Read the model definition and answer for the solid it produces. Units are mm, in the model's axes. Face numbers are marked on the shaded views. A direction names the side the tool comes from. Give positions to 0.01 mm unless a question says otherwise; leave off trailing zeros. Loops run counter-clockwise (first coordinate to the right, second up) from the corner with the lowest first, then second, coordinate; pieces in that order, holes last. Notation, with made-up numbers: (-21, -9) - (28, -9) arc R24 cw to (28, 28) - close; hole circle Ø1 at (74, 85). An arc over 180 degrees is marked (long way). Write item = value, one per line.
```python
from build123d import *

# Parameters (mm, degrees)
SKETCH_2_OUTSIDE_W       = 102.04
SKETCH_2_OUTSIDE_H       = 102.04
SKETCH_2_OUTSIDE_W_2     = 32
SKETCH_2_OUTSIDE_H_2     = 32
CUT_EXTRUDE_1_DEPTH      = 24
CUT_EXTRUDE_2_DEPTH      = 5
CUT_EXTRUDE_3_DEPTH      = 243.590189414
CUT_EXTRUDE_3_DEPTH_BACK = 243.590189414
SKETCH_4_R               = 6


with BuildPart() as part:
    # Эскиз1 → Повернуть1 (revolve)
    with BuildSketch(Plane.XY, mode=Mode.PRIVATE) as revolve_1_sk:
        Polygon((0, 0), (0, 19), (-1, 20), (-160, 20), (-160, 25), (-184, 25), (-184, 16), (-239, 16), (-240, 15), (-240, 0), align=None)
    revolve(revolve_1_sk.sketch.rotate(Axis((-178.322580645, 0, 0), (1, 0, 0)), 90), axis=Axis((-178.322580645, 0, 0), (1, 0, 0)))

    # Эскиз2 outside → Вырез-Вытянуть1 (cut)
    with BuildSketch(Plane(origin=(-144, 0, 0), x_dir=(0, 0, -1), z_dir=(1, 0, 0))):
        Rectangle(SKETCH_2_OUTSIDE_W, SKETCH_2_OUTSIDE_H)
        Rectangle(SKETCH_2_OUTSIDE_W_2, SKETCH_2_OUTSIDE_H_2, mode=Mode.SUBTRACT)
    extrude(amount=CUT_EXTRUDE_1_DEPTH, mode=Mode.SUBTRACT)

    # Эскиз3 → Вырез-Вытянуть2 (cut)
    with BuildSketch(Plane(origin=(0, -16, 0), x_dir=(-1, 0, 0), z_dir=(0, -1, 0))):
        with BuildLine():
            Line((227, -6), (197, -6))
            ThreePointArc((197, -6), (191, 0), (197, 6))
            Line((197, 6), (227, 6))
            ThreePointArc((227, 6), (233, 0), (227, -6))
        make_face()
    extrude(amount=-CUT_EXTRUDE_2_DEPTH, mode=Mode.SUBTRACT)

    # Эскиз4 → Вырез-Вытянуть3 (cut, two sides: drawn at the far end of the back side and taken through both)
    with BuildSketch(Plane(origin=(0, 0, 0), x_dir=(-1, 0, 0), z_dir=(0, -0.7071067811865488, 0.7071067811865464)).offset(-CUT_EXTRUDE_3_DEPTH_BACK)):
        with Locations(Location((24, 0, 0), (0, 0, 90))):
            Circle(SKETCH_4_R)
    extrude(amount=CUT_EXTRUDE_3_DEPTH + CUT_EXTRUDE_3_DEPTH_BACK, mode=Mode.SUBTRACT)


solid = part.part
```
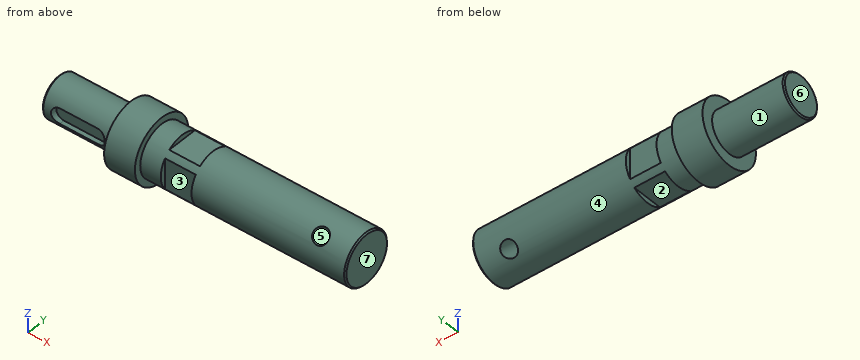
1) A tool of negligible diameter and unlimited length cuts with its end or side. For the marked faces 1, 2, 3 and 4, from which of +Z, -Z, +X, -X, +Y, -Y can it reach the whole face along a straight path? Write none if from no direction.
Output:
face_1 = -X
face_2 = -Z, +Y, -Y
face_3 = +Z, -Z, -Y
face_4 = +X
2) Find the intervals of material crossed by probe 1 along X at (y, z) = (-17.5, 7); probe 2 along X at (y, z) = (-14, 0); probe 3 along Z at (x, y) = (-97, 1), in increasing order.
Output:
probe_1 = -184 to -144, -120 to 0
probe_2 = -240 to -233, -191 to 0
probe_3 = -19.97 to 19.97
3) A cutting plane is placed at B-B on x = -77.5. Determine the outline of the cut face in (y, z), then the cut area to 3 significant figures.
Output:
outline = circle Ø40 at (0, 0)
area = 1,260 mm²
4) The mould has two halves that part along X. Classify the marked faces 5, 6 and 7: pulls with the +X half, pulls with the -X half, needs draft (parallel to the pull), parting line crosses it, or undercut.
Output:
face_5 = undercut
face_6 = pulls with the -X half
face_7 = pulls with the +X half
5) A cutting plane is placed at A-A on x = -122.5. Determine the outline of the cut face in (y, z).
Output:
outline = (-16, -12) arc R20 ccw to (-12, -16) - (12, -16) arc R20 ccw to (16, -12) - (16, 12) arc R20 ccw to (12, 16) - (-12, 16) arc R20 ccw to (-16, 12) - close
6) Each of these flat-tipped pins is pushed along its axis until it touches: P1, Ø6, axis at x = -166, z = -6, coming from the +Y side; P2, Ø1.9, axis at x = -219, y = -13.5, coming from the -Z side; P3, Ø4, axis at x = -144.5, z = 11.5, coming from the +Y side. Where does it stop, or does it pass through?
Output:
P1 = 24.82
P2 = -9.92
P3 = 17.6
